Input: part model. Units: mm. Frame: model coordinates. Face numbers are marked on the shaded views. A direction names the side the tool comes from. Round coordinates to 2 decimals unless told otherwise and drop trailing zeros. Loops run counter-clockwise (first coordinate to the right, second up) from the corner with the lowest first, then second, coordinate; pieces in that order, holes last.
1) Section A-A, the plane x = 0. Return loops of the section in (y, z), and give its area (3 significant figures).
2) Section C-C, the plane z = 5.75. Return loops of the section in (x, y), and give its area (3 significant figures).
3) Section D-D, the plane z = 1.5. Return loops of the section in (x, y).
4) First-contact query: pin 1 (2 mm diameter, centred on x = 6, z = 1.5, fed in from +Y); pin 2 (8 mm diameter, centred on x = -4, y = -4.5, fed in from -Z); pin 3 (1 mm diameter, centred on x = -3.5, z = 5.5, fed in from -Y); pin 4 (2 mm diameter, centred on x = -6, z = 1, fed in from -Y). Flat tips, straight axial feed; report the tip coordinate or a pass-through.
5) Ray query, line 1 along Z through (x, y) = (-1.25, -3.25); line 2 along X through (y, z) = (0.5, 2); line 3 along X through (y, z) = (6.25, 3.75). Return the intervals inside material, ascending.
6) Access query for the marked faces 1 and 2. Directions: +Z, -Z, +X, -X, +Y, -Y. A direction counts if a zero-diameter tool reaches every point of the face in a straight line with its end or side. Return the directions, or none.
from build123d import *

# Parameters (mm, degrees)
SKETCH_R     = 8.2
PAD_DEPTH    = 4.5
SKETCH001_R  = 2.5
PAD001_DEPTH = 4
FILLET_R     = 1


with BuildPart() as part:
    # Sketch → Pad (new body)
    with BuildSketch(Plane.XY):
        Circle(SKETCH_R)
    extrude(amount=PAD_DEPTH)

    # Sketch001 (on Face3 of Pad) → Pad001 (join)
    with BuildSketch(Plane.XY.offset(4.5)):
        Circle(SKETCH001_R)
    extrude(amount=PAD001_DEPTH)

    # Fillet
    fillet_edges = [part.edges().sort_by_distance(p)[0] for p in [
        (-8.2, 0, 4.5),
    ]]
    fillet(fillet_edges, radius=FILLET_R)


solid = part.part
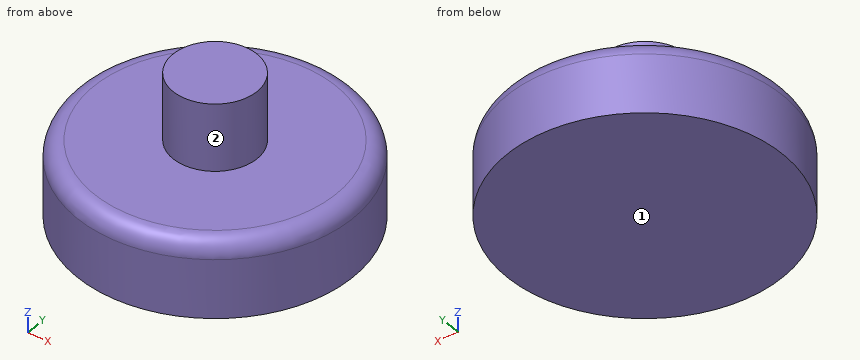
Final values:
1. outline: (-8.2, 0) - (8.2, 0) - (8.2, 3.5) arc R1 ccw to (7.2, 4.5) - (2.5, 4.5) - (2.5, 8.5) - (-2.5, 8.5) - (-2.5, 4.5) - (-7.2, 4.5) arc R1 ccw to (-8.2, 3.5) - close
1. area: 93.4 mm2
2. outline: circle Ø5 at (0, 0)
2. area: 19.6 mm2
3. outline: circle Ø16.4 at (0, 0)
4. pin 1: stops at y = 6.5
4. pin 2: stops at z = 0
4. pin 3: passes through
4. pin 4: stops at y = -6.5
5. line 1: z = 0 to 4.5
5. line 2: x = -8.18 to 8.18
5. line 3: x = -5.26 to 5.26
6. face 1: -Z, +X, -X, +Y, -Y
6. face 2: +Z
